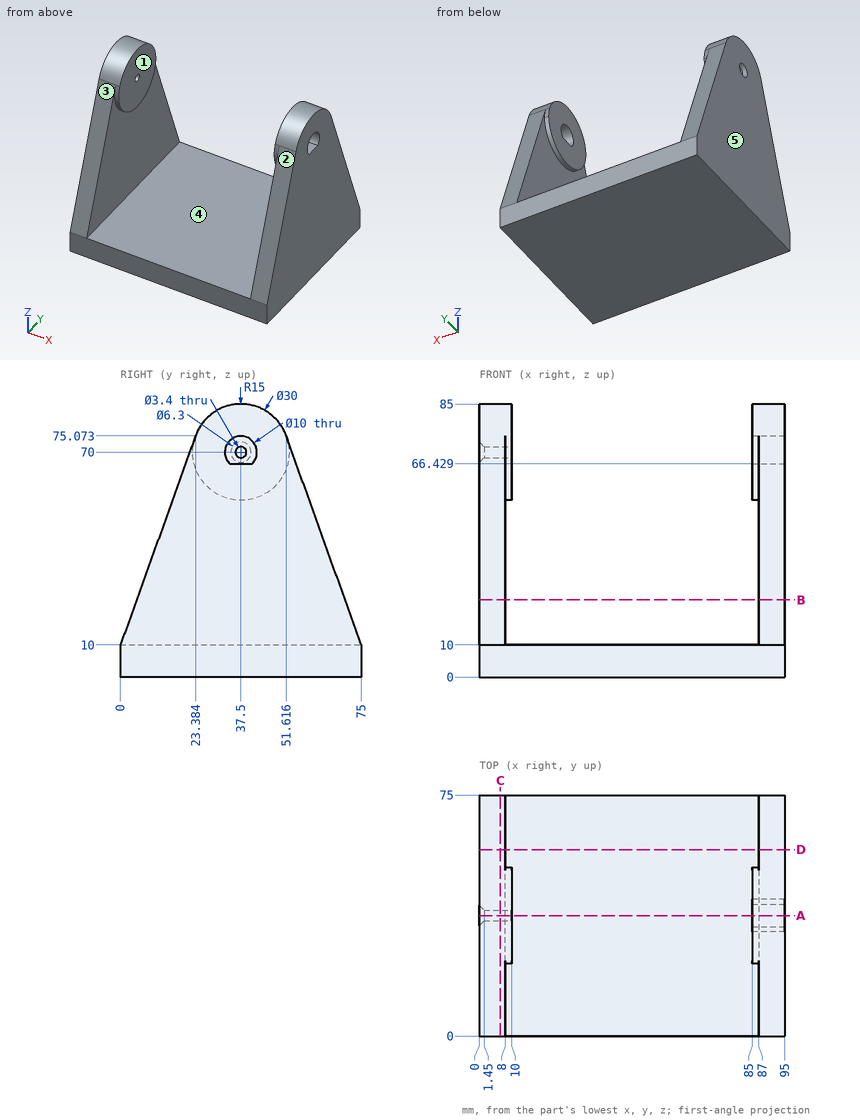
Print and shaded views of the part. All mm, measured from the part's lowest x, y and z. A direction names the side the tool comes from. Round coordinates to 2 decimals unless told otherwise and drop trailing zeros. Order: outer loops, then holes, each group sorted by start corner. A loop starts at its lowest first (then second) coordinate and runs counter-clockwise, first axis right, second up.
Q1. Slice it at A-A (y = 37.5). Write the cut outline in (x, z), and give its area (3 significant figures).
Q2. Wall check: L1, parallel to X at y = 66.5, z = 28.5; L2, parallel to Z at x = 10.5, y = 26; L3, parallel to X at y = 52, z = 70. Give the ranges that are in metal, low to high.
Q3. Which spindle directions (+Z, -Z, +X, -X, +Y, -Y) get a long thin tool onto all of the face, cutting with end or side? Do the marked faces 1 and 2. Say none if no direction does.
Q4. Two-plate mould, pull along X, no slides. Class the marked faces 3, 4 and 5: pulls with the +X half, pulls with the -X half, needs draft (parallel to the pull), parting line crosses it, or undercut.
Q5. Slice it at D-D (y = 58). Write the cut outline in (x, z).
Q6. Slice it at B-B (z = 24). Write the cut outline in (x, y), and give its area (3 significant figures).
Q7. Drop flat-ended pins along their axis: pin 1 (4 mm diameter, centred on y = 37.5, z = 70, fed in from +X); pin 2 (12 mm diameter, centred on x = 81.5, z = 42, fed in from +Y); pin 3 (3 mm diameter, centred on x = 15.5, y = 28, fed in from +Z). Give the stop position or say it passes through.
Q8. Slice it at C-C (x = 6.5). Write the cut outline in (y, z), and give its area (3 significant figures).
Results below:
1. outline: (0, 0) - (95, 0) - (95, 66.43) - (85, 66.43) - (85, 55) - (87, 55) - (87, 10) - (8, 10) - (8, 55) - (10, 55) - (10, 68.3) - (1.45, 68.3) - (0, 66.85) - close; (0, 73.15) - (1.45, 71.7) - (10, 71.7) - (10, 85) - (0, 85) - close; (85, 75) - (95, 75) - (95, 85) - (85, 85) - close
1. area: 2,150 mm2
2. L1: x = 0 to 8, 87 to 95
2. L2: z = 0 to 10
2. L3: x = 0 to 10, 85 to 95
3. face 1: +Z, +Y, -Y
3. face 2: +Z, +X, -X, -Y
4. face 3: needs draft
4. face 4: undercut
4. face 5: pulls with the -X half
5. outline: (0, 0) - (95, 0) - (95, 57.31) - (87, 57.31) - (87, 10) - (8, 10) - (8, 57.31) - (0, 57.31) - close
6. outline: (0, 5.03) - (8, 5.03) - (8, 69.97) - (0, 69.97) - close; (87, 5.03) - (95, 5.03) - (95, 69.97) - (87, 69.97) - close
6. area: 1,040 mm2
7. pin 1: stops at x = 10
7. pin 2: stops at y = 64.36
7. pin 3: stops at z = 10
8. outline: (0, 0) - (75, 0) - (75, 10) - (51.62, 75.07) arc R15 ccw to (23.38, 75.07) - (0, 10) - close; hole circle Ø3.4 at (37.5, 70)
8. area: 4,300 mm2
